Geometry check sheet. Reference: the model listing, model coordinates, mm. A direction names the side the tool comes from. Coordinates: 2 decimals unless noted, no trailing zeros. Order: outer loops, then holes, each group sorted by start corner. A loop starts at its lowest first (then second) coordinate and runs counter-clockwise, first axis right, second up.
```python
from build123d import *

# Parameters (mm, degrees)
SKETCH_1_R                     = 27.218239916
EXTRUDE_1_DEPTH                = 50
SPLIT_BODIES_1_SURFACE_1_BACK  = 231.852
SPLIT_BODIES_1_SURFACE_1_DEPTH = 463.704
SPLIT_BODIES_1_SURFACE_2_BACK  = 231.852
SPLIT_BODIES_1_SURFACE_2_DEPTH = 463.704


with BuildPart() as part:
    # 草图1 → 凸台-拉伸1 (new, symmetric)
    with BuildSketch(Plane.XY):
        with Locations((126.841, 106.1775)):
            Circle(SKETCH_1_R)
        with BuildLine():
            Line((36.476006197, 29.147891414), (56.67204093, 43.504108875))
            Line((56.67204093, 43.504108875), (56.67204093, 93.307484045))
            Line((56.67204093, 93.307484045), (92.496172884, 93.307484045))
            ThreePointArc((92.496172884, 93.307484045), (88.507151815, 108.556758389), (81.393508143, 122.622629526))
            ThreePointArc((81.393508143, 122.622629526), (81.328816917, 131.844883349), (89.661, 135.798220622))
            Line((89.661, 135.798220622), (152.57565846, 127.931864381))
            ThreePointArc((152.57565846, 127.931864381), (156.589044848, 125.482703859), (157.411382406, 120.853511867))
            Line((157.411382406, 120.853511867), (139.303205185, 49.257428232))
            Line((139.303205185, 49.257428232), (123.353516134, 49.257428232))
            Line((123.353516134, 49.257428232), (117.072161438, 27.122156161))
            Line((117.072161438, 27.122156161), (134.529857437, 27.122156161))
            Line((134.529857437, 27.122156161), (144.001, 0))
            Line((144.001, 0), (0, 0))
            Line((0, 0), (0, 29.147891414))
            Line((0, 29.147891414), (36.476006197, 29.147891414))
        make_face()
    extrude(amount=EXTRUDE_1_DEPTH, both=True)


with BuildPart() as body_2:
    # Split Bodies 1: the piece behind the surface
    add(part.part)
    # Split Bodies 1 surface: a surface, the sketch's curves swept straight by 463.704 mm
    with BuildLine(Plane.XY.offset(50).offset(-SPLIT_BODIES_1_SURFACE_1_BACK), mode=Mode.PRIVATE) as split_bodies_1_surface_1_path:
        Line((123.353516134, 49.257428232), (56.67204093, 49.257428232))
    split_bodies_1_surface_1 = Shell.extrude(split_bodies_1_surface_1_path.wire(), (0 * SPLIT_BODIES_1_SURFACE_1_DEPTH, 0 * SPLIT_BODIES_1_SURFACE_1_DEPTH, 1 * SPLIT_BODIES_1_SURFACE_1_DEPTH))
    split(bisect_by=split_bodies_1_surface_1, keep=Keep.BOTTOM)


with BuildPart() as part_1:
    add(part.part)

    # Split Bodies 1: split by a surface, the side it looks to stays
    # Split Bodies 1 surface: a surface, the sketch's curves swept straight by 463.704 mm
    with BuildLine(Plane.XY.offset(50).offset(-SPLIT_BODIES_1_SURFACE_2_BACK), mode=Mode.PRIVATE) as split_bodies_1_surface_2_path:
        Line((123.353516134, 49.257428232), (56.67204093, 49.257428232))
    split_bodies_1_surface_2 = Shell.extrude(split_bodies_1_surface_2_path.wire(), (0 * SPLIT_BODIES_1_SURFACE_2_DEPTH, 0 * SPLIT_BODIES_1_SURFACE_2_DEPTH, 1 * SPLIT_BODIES_1_SURFACE_2_DEPTH))
    split(bisect_by=split_bodies_1_surface_2, keep=Keep.TOP)


solid = part_1.part
```
Item 1: Release check for a two-part mould opening along Y. For faces 3 (the face through (120.257, 38.345, 0.7)), 4 (the face through (46.4, 36.2, 0.7)), 5 (the face through (126, 27.122, 1)), 6 (the face through (56.672, 46, 1)) record: pulls with the +Y half, pulls with the -Y half, needs draft (parallel to the pull), parting line crosses it, or undercut.
Item 2: Sectioned sample at A-A (z = -8). Record the cut outline in (x, y), and give its area (3 significant figures).
Item 3: Sectioned sample at B-B (y = 12). Record the cut outline in (x, z), and give its area (3 significant figures).
Item 4: Sectioned sample at C-C (x = 29). Record the cut outline in (y, z).
Item 5: Tool access check on faces 1 (the face through (0, 14, 1)), 2 (the face through (18, 29.148, 1)). Record the directions out of +Z, -Z, +X, -X, +Y, -Y that give a thin tool (end or side, any length) a straight path to the whole face; none if there is none.
Item 6: Thickness scan on line 1 along Y through (x, z) = (35.5, 40.5); line 2 along Y through (x, z) = (130, 37); line 3 along X through (y, z) = (29, 37.5). Record the ranges inside material, lowest first.
Item 7: Depth check by flat-ended pin: P1, Ø1.5, axis at y = 33.5, z = -9.5, coming from the -X side; P2, Ø6, axis at y = 41, z = -37, coming from the -X side; P3, Ø4.5, axis at y = 46.5, z = -3.5, coming from the -X side. Enter the tip coordinate at first touch or a pass-through.
Geometry check:
1. face 3: undercut
1. face 4: pulls with the +Y half
1. face 5: undercut
1. face 6: needs draft
2. outline: (0, 0) - (144, 0) - (134.53, 27.12) - (117.07, 27.12) - (123.35, 49.26) - (56.67, 49.26) - (56.67, 43.5) - (36.48, 29.15) - (0, 29.15) - close
2. area: 5,440 mm2
3. outline: (0, -50) - (139.81, -50) - (139.81, 50) - (0, 50) - close
3. area: 14,000 mm2
4. outline: (0, -50) - (29.15, -50) - (29.15, 50) - (0, 50) - close
5. face 1: +Z, -Z, -X, +Y, -Y
5. face 2: +Z, -Z, -X, +Y
6. line 1: y = 0 to 29.15
6. line 2: y = 0 to 27.12
6. line 3: x = 0 to 117.61
7. P1: stops at x = 41.54
7. P2: stops at x = 48.93
7. P3: stops at x = 56.67
